```python
from build123d import *

# Parameters (mm, degrees)
F1_DEPTH = 120
F3_R     = 3.875
F4_DEPTH = 8
F2_R     = 3.875
F5_DEPTH = 8


with BuildPart() as f1:
    # F0 (on Front) → F1 (new body, symmetric)
    with BuildSketch(Plane.XZ):
        with BuildLine():
            Line((3, 4), (-3, 4))
            ThreePointArc((-3, 4), (0, -5), (3, 4))
        make_face()
    extrude(amount=F1_DEPTH, both=True)

    # F3 (on face) → F4 (join)
    with BuildSketch(Plane.XZ.offset(120)):
        Circle(F3_R)
    extrude(amount=F4_DEPTH)

    # F2 (on face) → F5 (join)
    with BuildSketch(Plane(origin=(0, 120, 0), x_dir=(-1, 0, 0), z_dir=(0, 1, 0))):
        Circle(F2_R)
    extrude(amount=F5_DEPTH)


solid = f1.part
```
The listing builds one solid part. Answer for the finished solid, in the listing's coordinates (mm). A direction names the side the tool comes from. Coordinates: 2 decimals unless noted, no trailing zeros. Loops run counter-clockwise (first coordinate to the right, second up) from the corner with the lowest first, then second, coordinate; pieces in that order, holes last. Notation, with made-up numbers: (-9.5, 8.5) - (13.5, 8.5) arc R37 cw to (13.5, 46.5) - close; hole circle Ø4 at (40.5, -27.5). An arc over 180 degrees is marked (long way). Use a Markdown table: item, result. Add a question column.
1) The part is cut by section B-B, the plane x = 1. Give the vertices of the cut face in (y, z), and give its area (3 significant figures).
2) The part is cut by section A-A, the plane z = -2.25. Give the vertices of the cut face in (x, y), and give its area (3 significant figures).
3) Find the intervals of material crossed by line 1 (Z direction, x = -0.5, y = 70.5); line 2 (X direction, y = -64.5, z = -4); line 3 (Y direction, x = -0.5, z = -4.25), in increasing order.
4) The part is cut by section C-C, the plane y = -100. Give the vertices of the cut face in (x, z), and give its area (3 significant figures).
5) For faces 1 (the cylindrical face through (0.504, 123.944, 3.842)), 2 (the flat face through (0, 128, 0)), 3 (the flat face through (-1, -120, -4)), determine the directions among +Z, -Z, +X, -X, +Y, -Y from which every point of the face is accessible in a straight line to the end or side of a thin tool.
6) Given pin 1 (5 mm diameter, centred on y = -18.5, z = -3.5, fed in from -X), flat-ended and moving along its own axis, determine where the tip first touches the part or whether it passes through.
Here are the results:
| question | item | result |
|---|---|---|
| 1 | outline | (-128, -3.74) - (-120, -3.74) - (-120, -4.9) - (120, -4.9) - (120, -3.74) - (128, -3.74) - (128, 3.74) - (120, 3.74) - (120, 4) - (-120, 4) - (-120, 3.74) - (-128, 3.74) - close |
| 1 | area | 2,260 mm^2 |
| 2 | outline | (-4.47, -120) - (-3.15, -120) - (-3.15, -128) - (3.15, -128) - (3.15, -120) - (4.47, -120) - (4.47, 120) - (3.15, 120) - (3.15, 128) - (-3.15, 128) - (-3.15, 120) - (-4.47, 120) - close |
| 2 | area | 2,240 mm^2 |
| 3 | line 1 | z = -4.97 to 4 |
| 3 | line 2 | x = -3 to 3 |
| 3 | line 3 | y = -120 to 120 |
| 4 | outline | (-3, 4) arc R5 ccw (long way) to (3, 4) - close |
| 4 | area | 74.5 mm^2 |
| 5 | face 1 | +Y |
| 5 | face 2 | +Z, -Z, +X, -X, +Y |
| 5 | face 3 | -Y |
| 6 | pin 1 | stops at x = -4.9 |
